Geometry check sheet. Reference: the model listing, model coordinates, mm. A direction names the side the tool comes from. Coordinates: 2 decimals unless noted, no trailing zeros. Write each loop counter-clockwise with the first axis right and the second up, starting at its lowest first coordinate (ties: lowest second). Pieces come first, ordered by that corner, then holes. Notation, with made-up numbers: (59, -22.75) - (63, -22.75) arc R20 ccw to (63, -16.75) - close; hole circle Ø2 at (16.5, -37). An arc over 180 degrees is marked (long way). Answer as a JSON object with one key per item and string values. Group by question number.
from build123d import *

# Parameters (mm, degrees)
F1_DEPTH = 16.256
F2_R     = 5.08
F3_W     = 70.9863193333
F3_H     = 35.4931587353
F4_DEPTH = 33.02
F5_R     = 7.3585229381
F7_D     = 6.35
F7_DEPTH = 16.9956048409


with BuildPart() as f1:
    # F0 (on Top) → F1 (new body)
    with BuildSketch(Plane.XY):
        with BuildLine():
            Line((57.6345990729, 28.3577627349), (-45.6030252707, 28.3577627349))
            ThreePointArc((-45.6030252707, 28.3577627349), (-49.1951277191, 26.8698651833), (-50.6830252707, 23.2777627349))
            Line((-50.6830252707, 23.2777627349), (-50.6830252707, -11.9146048409))
            ThreePointArc((-50.6830252707, -11.9146048409), (-49.1951277191, -15.5067072893), (-45.6030252707, -16.9946048409))
            Line((-45.6030252707, -16.9946048409), (57.6345990729, -16.9946048409))
            ThreePointArc((57.6345990729, -16.9946048409), (61.2267015214, -15.5067072893), (62.7145990729, -11.9146048409))
            Line((62.7145990729, -11.9146048409), (62.7145990729, 23.2777627349))
            ThreePointArc((62.7145990729, 23.2777627349), (61.2267015214, 26.8698651833), (57.6345990729, 28.3577627349))
        make_face()
    extrude(amount=F1_DEPTH)

    # F2
    f2_edges = [f1.edges().sort_by_distance(p)[0] for p in [
        (-49.195128, -15.506707, 16.256),
    ]]
    fillet(f2_edges, radius=F2_R)

    # F3 (on Top) → F4 (join)
    with BuildSketch(Plane.XY):
        with Locations((5.5646058172, 5.8653946035)):
            Rectangle(F3_W, F3_H)
    extrude(amount=F4_DEPTH)

    # F5
    f5_edges = [f1.edges().sort_by_distance(p)[0] for p in [
        (5.564606, 23.611974, 33.02),
        (-29.928554, 5.865395, 33.02),
        (5.564606, -11.881185, 33.02),
        (41.057765, 5.865395, 33.02),
    ]]
    fillet(f5_edges, radius=F5_R)

    # F7 (through all, one way)
    with BuildSketch(Plane(origin=(0, 0, 0), x_dir=(1, 0, 0), z_dir=(0, 1, 0))):
        with Locations((53.6909215152, -3.4590789583), (-42.2609224916, -3.4590789583)):
            Circle(F7_D / 2)
    extrude(amount=-F7_DEPTH, mode=Mode.SUBTRACT)


solid = f1.part
(1) Set-up check for faces 1 (the face through (5, -11.881, 21)), 2 (the face through (-29.929, 6, 21)), 3 (the face through (5, 23.612, 21)): record each of +Z, -Z, +X, -X, +Y, -Y from which the full face is reachable in a straight line by a thin tool's end or side.
(2) Gauge pin test, flat ends, axial feed: pin 1 (1.5 mm diameter, centred on y = -10.5, z = 26, fed in from -X); pin 2 (10.5 mm diameter, centred on y = 1.5, z = 19, fed in from -X); pin 3 (1.9 mm diameter, centred on x = 53, z = 3.5, fed in from -Y). Record the tip position at first contact, or that the pin passes through.
(3) Section check C-C (y = -8). Record the cut outline in (x, z) (3 decimals).
(4) Section check B-B (x = 17.5). Record the cut outline in (y, z) (3 decimals), and give its area (3 significant figures).
(5) Draft check along X on faces 4 (the face through (41.058, 6, 21)), 5 (the face through (7, 28.358, 6)), 6 (the face through (54, 0, 3)). Enter one of: +X half, -X half, draft (parallel to the pull), parting line (faces both ways), or undercut.
(6) Section check D-D (z = 14). Record the cut outline in (x, y), and give its area (3 significant figures).
(7) Section check A-A (y = 12.5). Record the cut outline in (x, z).
(8) Material ranges on L1, parallel to X at y = -7.5, z = 4; L2, parallel to X at y = 13.5, z = 22; L3, parallel to X at y = 23, z = 26, recorded low to high. Write a range as [from, to].
Conclusion:
{
 "1": {"face 1": "+Z, +X, -X, -Y", "face 2": "+Z, -X, +Y, -Y", "face 3": "+Z, +X, -X, +Y"},
 "2": {"pin 1": "stops at x = -29.93", "pin 2": "stops at x = -49.98", "pin 3": "stops at y = 0"},
 "3": {"outline": "(-50.683, 0) - (62.715, 0) - (62.715, 11.176) arc R5.08 ccw to (57.635, 16.256) - (41.058, 16.256) - (41.058, 25.661) arc R7.359 ccw to (37.177, 32.147) - (-26.047, 32.147) arc R7.359 ccw to (-29.929, 25.661) - (-29.929, 16.256) - (-45.603, 16.256) arc R5.08 ccw to (-50.683, 11.176) - close; hole circle Ø6.35 at (-42.261, 3.459); hole circle Ø6.35 at (53.691, 3.459)"},
 "4": {"outline": "(-16.995, 0) - (28.358, 0) - (28.358, 11.176) arc R5.08 ccw to (23.612, 16.245) - (23.612, 25.661) arc R7.359 ccw to (16.253, 33.02) - (-4.523, 33.02) arc R7.359 ccw to (-11.881, 25.661) - (-11.881, 16.256) - (-11.915, 16.256) arc R5.08 ccw to (-16.995, 11.176) - close", "area": "1,300 mm^2"},
 "5": {"face 4": "+X half", "face 5": "draft", "face 6": "undercut"},
 "6": {"outline": "(-49.83, -11.91) arc R4.22 ccw to (-45.6, -16.14) - (57.63, -16.14) arc R4.22 ccw to (61.86, -11.91) - (61.86, 23.28) arc R4.22 ccw to (57.63, 27.5) - (-45.6, 27.5) arc R4.22 ccw to (-49.83, 23.28) - close", "area": "4,860 mm^2"},
 "7": {"outline": "(-50.68, 0) - (62.71, 0) - (62.71, 11.18) arc R5.08 ccw to (57.63, 16.26) - (41.06, 16.26) - (41.06, 25.66) arc R7.36 ccw to (33.7, 33.02) - (-22.57, 33.02) arc R7.36 ccw to (-29.93, 25.66) - (-29.93, 16.26) - (-45.6, 16.26) arc R5.08 ccw to (-50.68, 11.18) - close"},
 "8": {"L1": "x = [-50.68, -45.39], [-39.13, 50.56], [56.82, 62.71]", "L2": "x = [-29.93, 41.06]", "L3": "x = [-29.92, 41.05]"}
}
